Autodesk Fusion 360 part; units mm, degrees
sketch "Sketch1" plane through (0, 0, 0) normal (0, 0, 1) x (1, 0, 0)
  circle A0 centre (0, 0) radius 11.25
  dimension "d1" = 22.5
extrude "Extrude1" add sketch "Sketch1" along normal blind 21 makes body 1
sketch "Sketch2" plane through (0, 0, 0) normal (0, 0, 1) x (1, 0, 0)
  line L0 (-10, 1) -> (10, 1)
  line L1 (10, 1) -> (10, -1)
  line L2 (10, -1) -> (-10, -1)
  line L3 (-10, -1) -> (-10, 1)
extrude "Extrude2" add sketch "Sketch2" along normal blind 121 separate body makes body 2
sketch "Sketch3" plane through (0, 0, 0) normal (0, 0, 1) x (1, 0, 0)
  line L0 (-1, 10) -> (1, 10)
  line L1 (1, 10) -> (1, -10)
  line L2 (1, -10) -> (-1, -10)
  line L3 (-1, -10) -> (-1, 10)
extrude "Extrude3" add sketch "Sketch3" along normal blind 121 separate body makes body 3
sketch "Sketch5" plane through (0, 0, 0) normal (0, 1, 0) x (1, 0, 0)
  line L0 (0, -123) -> (11, -123)
  line L1 (11, -123) -> (11, -100)
  line L2 (11, -100) -> (1, -121)
  line L3 (1, -121) -> (0, -121)
  line L4 (0, -121) -> (0, -123)
revolve "Revolve1" cut sketch "Sketch5" angle 360 about axis through (0, 0, 1.75) along (0, 0, 1) bodies 2 3
sketch "Sketch6" plane through (0, 0, 0) normal (0, 0, 1) x (1, 0, 0)
  circle A0 centre (0, 0) radius 7
  dimension "d9" = 14
extrude "Extrude4" add 1 faces at (1.0392, -6.3884, 21) along direction (0, 0, 1) blind 3 on bodies 1 bodies 1 2 3
extrude "Extrude5" cut sketch "Sketch6" along normal blind 21 bodies 1
Input: part model. Units: mm. Frame: model coordinates. A direction names the side the tool comes from. Coordinates: 2 decimals unless noted, no trailing zeros. Write each loop counter-clockwise with the first axis right and the second up, starting at its lowest first coordinate (ties: lowest second). Pieces come first, ordered by that corner, then holes.
1) Section A-A on z = 67.5. Output: boundary loops of the cut face in (x, y).
2) Pin query (flat end, axial travel): pin 1 Ø10 at (y, z) = (5, 89.5) entering from -X; pin 2 Ø10 at (y, z) = (-7, 78.5) entering from +X; pin 3 Ø11 at (x, y) = (-3, 1.5) entering from -Z; pin 4 Ø12 at (x, y) = (-4, 8.5) entering from +Z. Return the tip coordinate at first contact, or that it passes through.
3) Section B-B on z = 19. Output: boundary loops of the cut face in (x, y), and give its area (3 significant figures).
4) Set-up query: faces 5 (the flat face through (6, -1, 71)), 6 (the flat face through (-1, 5, 71)), 7 (the cylindrical face through (6.466, 2.681, 10.353)), 8 (the flat face through (0, 10, 63)), 9 (the flat face through (0, -10, 63)). Return all of +Z, -Z, +X, -X, +Y, -Y with unobstructed straight access to the full face (end or side cutting, diameter ignored); none if empty.
5) Mould query, pull axis Y, two halves, no side actions, for faces 1 (the flat face through (-5, -1, 71)), 2 (the flat face through (2, -2, 24)), 3 (the flat face through (5, 1, 71)), 4 (the flat face through (0, 0, 21)). Classes: pulls with the +Y half, pulls with the -Y half, needs draft (parallel to the pull), parting line crosses it, or undercut.
6) Material intervals for line 1 along Y through (x, z) = (0, 7); line 2 along Y through (x, z) = (-7.75, 96.5); line 3 along Z through (x, y) = (-8.25, -2), sorted ascending.
Check result:
1. outline: (-10, -1) - (-1, -1) - (-1, -10) - (1, -10) - (1, -1) - (10, -1) - (10, 1) - (1, 1) - (1, 10) - (-1, 10) - (-1, 1) - (-10, 1) - close
2. pin 1: stops at x = -10
2. pin 2: stops at x = 1
2. pin 3: stops at z = 0
2. pin 4: stops at z = 115.85
3. outline: circle Ø22.5 at (0, 0); hole circle Ø14 at (0, 0)
3. area: 244 mm2
4. face 5: +Z, +X, -Y
4. face 6: +Z, -X, +Y
4. face 7: -Z
4. face 8: +Z, +X, -X, +Y
4. face 9: +Z, +X, -X, -Y
5. face 1: pulls with the -Y half
5. face 2: needs draft
5. face 3: pulls with the +Y half
5. face 4: undercut
6. line 1: y = -11.25 to -7, 7 to 11.25
6. line 2: y = -1 to 1
6. line 3: z = 0 to 24
